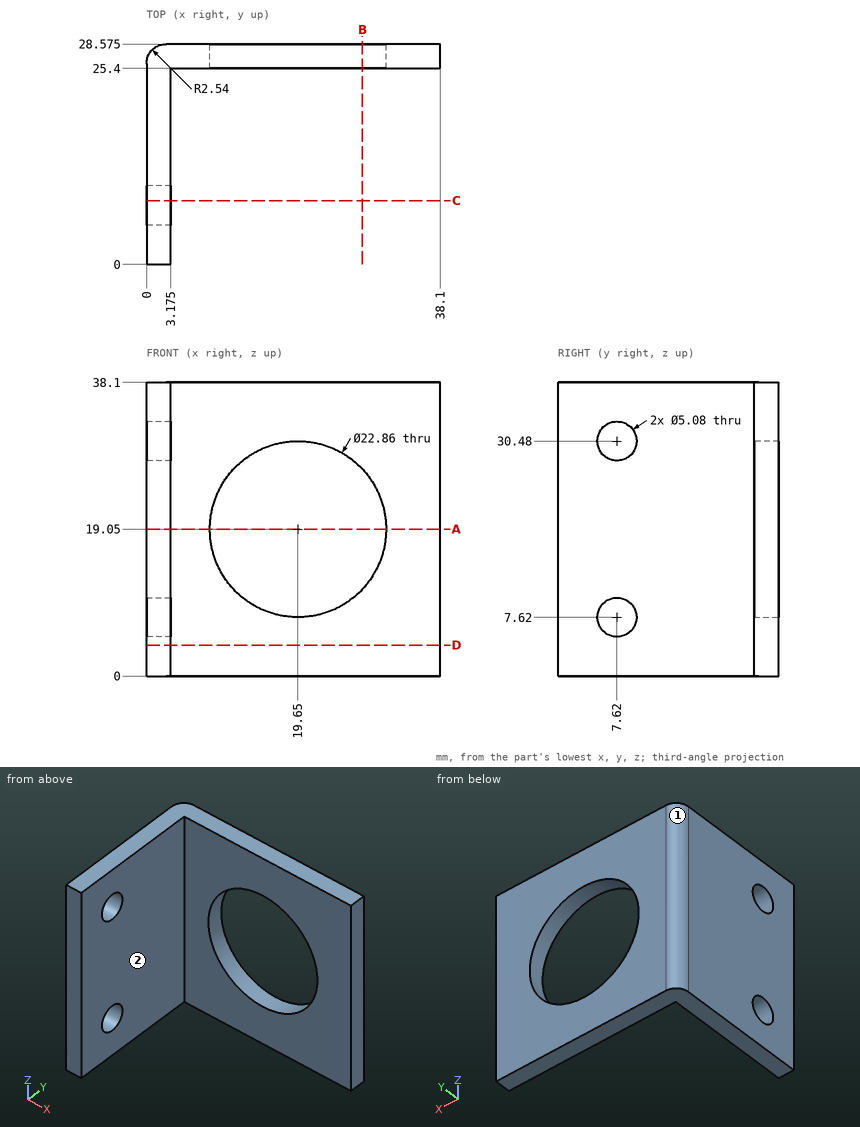
The figure shows three views and two pictorial views of one solid part (mm, origin at its lowest corner). Answer the questions. A direction names the side the tool comes from. Give positions to 0.01 mm unless a question says otherwise; leave off trailing zeros. Write each loop counter-clockwise with the first axis right and the second up, starting at its lowest first coordinate (ties: lowest second). Pieces come first, ordered by that corner, then holes. Notation, with made-up numbers: (-0.75, -27) - (42.25, -27) arc R20 cw to (42.25, -3) - close; hole circle Ø4 at (-1, -24). An arc over 180 degrees is marked (long way). Return JSON: item names as keys, results as strings.
Q1. A cutting plane is placed at B-B, the plane x = 28. Determine the outline of the cut face in (y, z) (3 decimals), and give its area (3 significant figures).
Reply:
{"outline": "(25.4, 0) - (28.575, 0) - (28.575, 11.245) - (25.4, 11.245) - close; (25.4, 26.855) - (28.575, 26.855) - (28.575, 38.1) - (25.4, 38.1) - close", "area": "71.4 mm²"}
Q2. A cutting plane is placed at C-C, the plane y = 8.25. Determine the outline of the cut face in (x, z) (1 decimal).
Reply:
{"outline": "(0, 0) - (3.2, 0) - (3.2, 5.2) - (0, 5.2) - close; (0, 10.1) - (3.2, 10.1) - (3.2, 28) - (0, 28) - close; (0, 32.9) - (3.2, 32.9) - (3.2, 38.1) - (0, 38.1) - close"}
Q3. A cutting plane is placed at A-A, the plane z = 19.05. Determine the outline of the cut face in (x, y) (3 decimals), and give its area (3 significant figures).
Reply:
{"outline": "(0, 0) - (3.175, 0) - (3.175, 25.4) - (8.22, 25.4) - (8.22, 28.575) - (2.54, 28.575) arc R2.54 ccw to (0, 26.035) - close; (31.08, 25.4) - (38.1, 25.4) - (38.1, 28.575) - (31.08, 28.575) - close", "area": "128 mm²"}
Q4. For the marked faces 1 and 2, determine the directions among +Z, -Z, +X, -X, +Y, -Y from which every point of the face is accessible in a straight line to the end or side of a thin tool.
Reply:
{"face 1": "+Z, -Z, -X, +Y", "face 2": "+Z, -Z, +X, -Y"}
Q5. A cutting plane is placed at D-D, the plane z = 4. Determine the outline of the cut face in (x, y) (3 decimals).
Reply:
{"outline": "(0, 0) - (3.175, 0) - (3.175, 25.4) - (38.1, 25.4) - (38.1, 28.575) - (2.54, 28.575) arc R2.54 ccw to (0, 26.035) - close"}
Q6. Consider line 1 along X through (y, z) = (3, 34.5) (3 decimals); line 2 along Y through (x, z) = (5.5, 32) (3 decimals); line 3 along Y through (x, z) = (1, 30.48) (1 decimal). Determine where each line is inside the solid, lowest interval first. Write a range as [from, to].
Reply:
{"line 1": "[0, 3.175]", "line 2": "[25.4, 28.575]", "line 3": "[0, 5.1], [10.2, 28.1]"}
Q7. Given P1, Ø7.5, axis at y = 15.5, z = 10, coming from the +X side (3 decimals); P2, Ø10.5, axis at x = 13.5, z = 27, coming from the -Y side, each flat-ended and moving along its own axis, determine where each tip first touches the part or whether it passes through.
Reply:
{"P1": "x = 3.175", "P2": "y = 25.4"}
